For this review, take the finished solid that the model builds, in its own axes (mm). Give positions to 0.01 mm unless a question says otherwise; leave off trailing zeros. Loops run counter-clockwise (first coordinate to the right, second up) from the corner with the lowest first, then second, coordinate; pieces in that order, holes last. Notation, with made-up numbers: (5.25, 53) - (11.25, 53) arc R21 cw to (11.25, 89) - close; hole circle Ø10 at (-10, 5). An arc over 180 degrees is marked (long way). Put each result on its own line as item: value.
from build123d import *

# Parameters (mm, degrees)
F0_W     = 25.4
F0_H     = 52.7300323124
F1_DEPTH = 2.54
F2_R     = 1.397
F3_DEPTH = 2.541
F5_DEPTH = 25.4


with BuildPart() as f1:
    # F0 (on Top) → F1 (new body)
    with BuildSketch(Plane.XY):
        with Locations((0, 24.4349838438)):
            Rectangle(F0_W, F0_H)
        with BuildLine():
            Line((4.318, 33.2232), (-4.318, 33.2232))
            ThreePointArc((-4.318, 33.2232), (-8.437248663, 31.516951337), (-6.731, 35.6362))
            Line((-6.731, 35.6362), (-6.731, 44.2722))
            ThreePointArc((-6.731, 44.2722), (-8.437248663, 48.391448663), (-4.318, 46.6852))
            Line((-4.318, 46.6852), (4.318, 46.6852))
            ThreePointArc((4.318, 46.6852), (6.731, 49.0982), (9.144, 46.6852))
            ThreePointArc((9.144, 46.6852), (8.437248663, 44.978951337), (6.731, 44.2722))
            Line((6.731, 44.2722), (6.731, 35.6362))
            ThreePointArc((6.731, 35.6362), (8.437248663, 34.929448663), (9.144, 33.2232))
            ThreePointArc((9.144, 33.2232), (6.731, 30.8102), (4.318, 33.2232))
        make_face(mode=Mode.SUBTRACT)
        with BuildLine():
            Line((12.7, -50.8), (12.7, -1.9300323124))
            Line((12.7, -1.9300323124), (-12.7, -1.9300323124))
            Line((-12.7, -1.9300323124), (-12.7, -50.8))
            ThreePointArc((-12.7, -50.8), (0, -63.5), (12.7, -50.8))
        make_face()
        with BuildLine():
            Line((4.318, -50.5452646249), (-4.318, -50.5452646249))
            ThreePointArc((-4.318, -50.5452646249), (-8.437248663, -52.2515132879), (-6.731, -48.1322646249))
            Line((-6.731, -48.1322646249), (-6.731, -39.4962646249))
            ThreePointArc((-6.731, -39.4962646249), (-8.437248663, -35.3770159619), (-4.318, -37.0832646249))
            Line((-4.318, -37.0832646249), (4.318, -37.0832646249))
            ThreePointArc((4.318, -37.0832646249), (6.731, -34.6702646249), (9.144, -37.0832646249))
            ThreePointArc((9.144, -37.0832646249), (8.437248663, -38.7895132879), (6.731, -39.4962646249))
            Line((6.731, -39.4962646249), (6.731, -48.1322646249))
            ThreePointArc((6.731, -48.1322646249), (8.437248663, -48.8390159619), (9.144, -50.5452646249))
            ThreePointArc((9.144, -50.5452646249), (6.731, -52.9582646249), (4.318, -50.5452646249))
        make_face(mode=Mode.SUBTRACT)
        with BuildLine():
            ThreePointArc((-6.731, -48.1322646249), (-5.024751337, -48.8390159619), (-4.318, -50.5452646249))
            Line((-4.318, -50.5452646249), (4.318, -50.5452646249))
            ThreePointArc((4.318, -50.5452646249), (5.024751337, -48.8390159619), (6.731, -48.1322646249))
            Line((6.731, -48.1322646249), (6.731, -39.4962646249))
            ThreePointArc((6.731, -39.4962646249), (5.024751337, -38.7895132879), (4.318, -37.0832646249))
            Line((4.318, -37.0832646249), (-4.318, -37.0832646249))
            ThreePointArc((-4.318, -37.0832646249), (-5.024751337, -38.7895132879), (-6.731, -39.4962646249))
            Line((-6.731, -39.4962646249), (-6.731, -48.1322646249))
        make_face()
        with BuildLine():
            ThreePointArc((-6.731, 35.6362), (-5.024751337, 34.929448663), (-4.318, 33.2232))
            Line((-4.318, 33.2232), (4.318, 33.2232))
            ThreePointArc((4.318, 33.2232), (5.024751337, 34.929448663), (6.731, 35.6362))
            Line((6.731, 35.6362), (6.731, 44.2722))
            ThreePointArc((6.731, 44.2722), (5.024751337, 44.978951337), (4.318, 46.6852))
            Line((4.318, 46.6852), (-4.318, 46.6852))
            ThreePointArc((-4.318, 46.6852), (-5.024751337, 44.978951337), (-6.731, 44.2722))
            Line((-6.731, 44.2722), (-6.731, 35.6362))
        make_face()
    extrude(amount=F1_DEPTH)

    # F2 (on face) → F3 (cut, through all)
    with BuildSketch(Plane.XY.offset(2.54)):
        with BuildLine():
            Line((-1.397, 0), (1.397, 0))
            ThreePointArc((1.397, 0), (0, 1.397), (-1.397, 0))
        make_face()
        with BuildLine():
            ThreePointArc((-1.397, 0), (0, -1.397), (1.397, 0))
            Line((1.397, 0), (-1.397, 0))
        make_face()
        with BuildLine():
            ThreePointArc((0.9878281733, -42.8264364516), (0, -42.4172646249), (-0.9878281733, -42.8264364516))
            Line((-0.9878281733, -42.8264364516), (0, -43.8142646249))
            Line((0, -43.8142646249), (0.9878281733, -42.8264364516))
        make_face()
        with BuildLine():
            Line((0, -43.8142646249), (-0.9878281733, -42.8264364516))
            ThreePointArc((-0.9878281733, -42.8264364516), (-1.397, -43.8142646249), (-0.9878281733, -44.8020927982))
            Line((-0.9878281733, -44.8020927982), (0, -43.8142646249))
        make_face()
        with BuildLine():
            Line((0.9878281733, -42.8264364516), (0, -43.8142646249))
            Line((0, -43.8142646249), (0.9878281733, -44.8020927982))
            ThreePointArc((0.9878281733, -44.8020927982), (1.2906597069, -44.3488733799), (1.397, -43.8142646249))
            ThreePointArc((1.397, -43.8142646249), (1.2906597069, -43.2796558699), (0.9878281733, -42.8264364516))
        make_face()
        with BuildLine():
            Line((0.9878281733, -44.8020927982), (0, -43.8142646249))
            Line((0, -43.8142646249), (-0.9878281733, -44.8020927982))
            ThreePointArc((-0.9878281733, -44.8020927982), (0, -45.2112646249), (0.9878281733, -44.8020927982))
        make_face()
        with Locations((0, 43.8142646249)):
            Circle(F2_R)
    extrude(amount=-F3_DEPTH, mode=Mode.SUBTRACT)

    # F4 (on face) → F5 (cut)
    with BuildSketch(Plane.XY.offset(2.54)):
        with BuildLine():
            ThreePointArc((1.397, 12.7), (-0.9878281733, 13.6878281733), (0, 11.303))
            ThreePointArc((0, 11.303), (0.9878281733, 11.7121718267), (1.397, 12.7))
        make_face()
        with BuildLine():
            ThreePointArc((1.397, -12.7), (0.9878281733, -11.7121718267), (0, -11.303))
            ThreePointArc((0, -11.303), (-0.9878281733, -13.6878281733), (1.397, -12.7))
        make_face()
    extrude(amount=-F5_DEPTH, mode=Mode.SUBTRACT)


solid = f1.part
1) Wall thickness on line 1 (X direction, y = 12.7, z = 1.55); line 2 (Y direction, x = 0.5, z = 1.1); line 3 (Y direction, x = -5.75, z = 1.45): over which ranges is each line inside the solid? List them lowest first.
Geometry check:
line 1: x = -12.7 to -1.4, 1.4 to 12.7
line 2: y = -63.49 to -45.12, -42.51 to -14, -11.4 to -1.3, 1.3 to 11.4, 14 to 42.51, 45.12 to 50.8
line 3: y = -62.12 to -52.75, -48.34 to -39.29, -34.88 to 31.02, 35.43 to 44.48, 48.89 to 50.8
2) Take a section at A-A on y = 0. State the section outline as (x, z) points, and give its area (3 significant figures).
Geometry check:
outline: (-12.7, 0) - (-1.4, 0) - (-1.4, 2.54) - (-12.7, 2.54) - close; (1.4, 0) - (12.7, 0) - (12.7, 2.54) - (1.4, 2.54) - close
area: 57.4 mm²
3) Insertion check: pin 1 Ø7.5 at (x, y) = (-6.73, 33.22) entering from -Z. The pin has a flat end and moves straight along its axis. Give the tip position at first contact, or say it passes through.
Geometry check:
pin 1: stops at z = 0
4) Take a section at C-C on x = 11. State the section outline as (y, z) points.
Geometry check:
outline: (-57.15, 0) - (50.8, 0) - (50.8, 2.54) - (-57.15, 2.54) - close
5) Draft analysis for pull direction X (two halves, no side actions). For faces 1 (the face through (0, -6, 0)), 2 (the face through (0.303, 1.364, 1.288)), 3 (the face through (-0.18, 45.2, 1.29)), 4 (the face through (-12.7, 1, 1)), state which applies: pulls with the +X half, pulls with the -X half, needs draft (parallel to the pull), parting line crosses it, or undercut.
Geometry check:
face 1: needs draft
face 2: undercut
face 3: undercut
face 4: pulls with the -X half
6) Take a section at B-B on z = 2.15. State how many separate pieces and enclosed holes the cut face has, and give its area (3 significant figures).
Geometry check:
separate pieces: 1
enclosed holes: 13
area: 2,660 mm²
